```python
from build123d import *

# Parameters (mm, degrees)
F1_DEPTH = 43.942
F2_DEPTH = 1.5875


with BuildPart() as f1:
    # F0 (on Front) → F1 (new body)
    with BuildSketch(Plane.XZ):
        with BuildLine():
            Line((-187.452, 109.982), (-187.452, -109.982))
            Line((-187.452, -109.982), (-100.33, -109.982))
            Line((-100.33, -109.982), (-87.630004, -109.982))
            Line((-87.630004, -109.982), (-0.060038, -109.982))
            ThreePointArc((-0.060038, -109.982), (0, -109.981677), (0.060038, -109.982))
            Line((0.060038, -109.982), (87.630004, -109.982))
            Line((87.630004, -109.982), (100.33, -109.982))
            Line((100.33, -109.982), (187.452, -109.982))
            Line((187.452, -109.982), (187.452, 109.982))
            Line((187.452, 109.982), (100.33, 109.982))
            Line((100.33, 109.982), (87.630004, 109.982))
            Line((87.630004, 109.982), (0.060038, 109.982))
            ThreePointArc((0.060038, 109.982), (0, 109.981677), (-0.060038, 109.982))
            Line((-0.060038, 109.982), (-87.630004, 109.982))
            Line((-87.630004, 109.982), (-100.33, 109.982))
            Line((-100.33, 109.982), (-187.452, 109.982))
        make_face()
    extrude(amount=F1_DEPTH)

    # F0 (on Front) → F2 (join)
    with BuildSketch(Plane.XZ):
        with BuildLine():
            Line((-187.452, 123.952), (-187.452, 109.982))
            Line((-187.452, 109.982), (-100.33, 109.982))
            Line((-100.33, 109.982), (-100.33, 123.952))
            Line((-100.33, 123.952), (-120.4341, 123.952))
            Line((-120.4341, 123.952), (-120.4341, 119.612701))
            Line((-120.4341, 119.612701), (-120.4341, 119.579099))
            ThreePointArc((-120.4341, 119.579099), (-122.428, 117.601929), (-124.4219, 119.579099))
            Line((-124.4219, 119.579099), (-124.4219, 123.952))
            Line((-124.4219, 123.952), (-160.5661, 123.952))
            Line((-160.5661, 123.952), (-160.5661, 119.612701))
            Line((-160.5661, 119.612701), (-160.5661, 119.579099))
            ThreePointArc((-160.5661, 119.579099), (-161.15005, 118.18595), (-162.543199, 117.602))
            Line((-162.543199, 117.602), (-162.576801, 117.602))
            ThreePointArc((-162.576801, 117.602), (-163.96995, 118.18595), (-164.5539, 119.579099))
            Line((-164.5539, 119.579099), (-164.5539, 123.952))
            Line((-164.5539, 123.952), (-187.452, 123.952))
        make_face()
        with BuildLine():
            Line((-187.452, -109.982), (-187.452, -123.952))
            Line((-187.452, -123.952), (-164.5539, -123.952))
            Line((-164.5539, -123.952), (-164.5539, -119.579099))
            ThreePointArc((-164.5539, -119.579099), (-162.56, -117.601929), (-160.5661, -119.579099))
            Line((-160.5661, -119.579099), (-160.5661, -119.612701))
            Line((-160.5661, -119.612701), (-160.5661, -123.952))
            Line((-160.5661, -123.952), (-124.4219, -123.952))
            Line((-124.4219, -123.952), (-124.4219, -119.579099))
            ThreePointArc((-124.4219, -119.579099), (-122.428, -117.601929), (-120.4341, -119.579099))
            Line((-120.4341, -119.579099), (-120.4341, -119.612701))
            Line((-120.4341, -119.612701), (-120.4341, -123.952))
            Line((-120.4341, -123.952), (-100.33, -123.952))
            Line((-100.33, -123.952), (-100.33, -109.982))
            Line((-100.33, -109.982), (-187.452, -109.982))
        make_face()
        with BuildLine():
            ThreePointArc((5.588, 115.509962), (3.951541, 111.618459), (0.060038, 109.982))
            Line((0.060038, 109.982), (87.630004, 109.982))
            Line((87.630004, 109.982), (87.630004, 123.952))
            Line((87.630004, 123.952), (67.5259, 123.952))
            Line((67.5259, 123.952), (67.5259, 119.579099))
            ThreePointArc((67.5259, 119.579099), (65.532, 117.601929), (63.5381, 119.579099))
            Line((63.5381, 119.579099), (63.5381, 119.612701))
            Line((63.5381, 119.612701), (63.5381, 123.952))
            Line((63.5381, 123.952), (27.3939, 123.952))
            Line((27.3939, 123.952), (27.3939, 119.579099))
            ThreePointArc((27.3939, 119.579099), (25.4, 117.601929), (23.4061, 119.579099))
            Line((23.4061, 119.579099), (23.4061, 119.612701))
            Line((23.4061, 119.612701), (23.4061, 123.952))
            Line((23.4061, 123.952), (5.588, 123.952))
            Line((5.588, 123.952), (5.588, 115.630038))
            ThreePointArc((5.588, 115.630038), (5.588323, 115.57), (5.588, 115.509962))
        make_face()
        with BuildLine():
            Line((187.452, -109.982), (100.33, -109.982))
            Line((100.33, -109.982), (100.33, -123.952))
            Line((100.33, -123.952), (120.4341, -123.952))
            Line((120.4341, -123.952), (120.4341, -119.612701))
            ThreePointArc((120.4341, -119.612701), (120.434029, -119.5959), (120.4341, -119.579099))
            ThreePointArc((120.4341, -119.579099), (122.428, -117.601929), (124.4219, -119.579099))
            Line((124.4219, -119.579099), (124.4219, -123.952))
            Line((124.4219, -123.952), (160.5661, -123.952))
            Line((160.5661, -123.952), (160.5661, -119.612701))
            ThreePointArc((160.5661, -119.612701), (160.566029, -119.5959), (160.5661, -119.579099))
            ThreePointArc((160.5661, -119.579099), (162.56, -117.601929), (164.5539, -119.579099))
            Line((164.5539, -119.579099), (164.5539, -123.952))
            Line((164.5539, -123.952), (187.452, -123.952))
            Line((187.452, -123.952), (187.452, -109.982))
        make_face()
        with BuildLine():
            Line((-87.630004, 123.952), (-87.630004, 109.982))
            Line((-87.630004, 109.982), (-0.060038, 109.982))
            ThreePointArc((-0.060038, 109.982), (-3.951541, 111.618459), (-5.588, 115.509962))
            ThreePointArc((-5.588, 115.509962), (-5.588323, 115.57), (-5.588, 115.630038))
            Line((-5.588, 115.630038), (-5.588, 123.952))
            Line((-5.588, 123.952), (-23.4061, 123.952))
            Line((-23.4061, 123.952), (-23.4061, 119.612701))
            ThreePointArc((-23.4061, 119.612701), (-23.406029, 119.5959), (-23.4061, 119.579099))
            ThreePointArc((-23.4061, 119.579099), (-25.4, 117.601929), (-27.3939, 119.579099))
            Line((-27.3939, 119.579099), (-27.3939, 123.952))
            Line((-27.3939, 123.952), (-63.5381, 123.952))
            Line((-63.5381, 123.952), (-63.5381, 119.612701))
            ThreePointArc((-63.5381, 119.612701), (-63.538029, 119.5959), (-63.5381, 119.579099))
            ThreePointArc((-63.5381, 119.579099), (-65.532, 117.601929), (-67.5259, 119.579099))
            Line((-67.5259, 119.579099), (-67.5259, 123.952))
            Line((-67.5259, 123.952), (-87.630004, 123.952))
        make_face()
        with BuildLine():
            Line((-0.060038, -109.982), (-87.630004, -109.982))
            Line((-87.630004, -109.982), (-87.630004, -123.952))
            Line((-87.630004, -123.952), (-67.5259, -123.952))
            Line((-67.5259, -123.952), (-67.5259, -119.579099))
            ThreePointArc((-67.5259, -119.579099), (-65.532, -117.601929), (-63.5381, -119.579099))
            Line((-63.5381, -119.579099), (-63.5381, -119.612701))
            Line((-63.5381, -119.612701), (-63.5381, -123.952))
            Line((-63.5381, -123.952), (-27.3939, -123.952))
            Line((-27.3939, -123.952), (-27.3939, -119.579099))
            ThreePointArc((-27.3939, -119.579099), (-25.4, -117.601929), (-23.4061, -119.579099))
            Line((-23.4061, -119.579099), (-23.4061, -119.612701))
            Line((-23.4061, -119.612701), (-23.4061, -123.952))
            Line((-23.4061, -123.952), (-5.588, -123.952))
            Line((-5.588, -123.952), (-5.588, -115.630038))
            ThreePointArc((-5.588, -115.630038), (-5.588323, -115.57), (-5.588, -115.509962))
            ThreePointArc((-5.588, -115.509962), (-3.951541, -111.618459), (-0.060038, -109.982))
        make_face()
        with BuildLine():
            Line((87.630004, -109.982), (0.060038, -109.982))
            ThreePointArc((0.060038, -109.982), (3.951541, -111.618459), (5.588, -115.509962))
            ThreePointArc((5.588, -115.509962), (5.588323, -115.57), (5.588, -115.630038))
            Line((5.588, -115.630038), (5.588, -123.952))
            Line((5.588, -123.952), (23.4061, -123.952))
            Line((23.4061, -123.952), (23.4061, -119.612701))
            ThreePointArc((23.4061, -119.612701), (23.406029, -119.5959), (23.4061, -119.579099))
            ThreePointArc((23.4061, -119.579099), (25.4, -117.601929), (27.3939, -119.579099))
            Line((27.3939, -119.579099), (27.3939, -123.952))
            Line((27.3939, -123.952), (63.5381, -123.952))
            Line((63.5381, -123.952), (63.5381, -119.612701))
            ThreePointArc((63.5381, -119.612701), (63.538029, -119.5959), (63.5381, -119.579099))
            ThreePointArc((63.5381, -119.579099), (65.532, -117.601929), (67.5259, -119.579099))
            Line((67.5259, -119.579099), (67.5259, -123.952))
            Line((67.5259, -123.952), (87.630004, -123.952))
            Line((87.630004, -123.952), (87.630004, -109.982))
        make_face()
        with BuildLine():
            Line((100.33, 123.952), (100.33, 109.982))
            Line((100.33, 109.982), (187.452, 109.982))
            Line((187.452, 109.982), (187.452, 123.952))
            Line((187.452, 123.952), (164.5539, 123.952))
            Line((164.5539, 123.952), (164.5539, 119.579099))
            ThreePointArc((164.5539, 119.579099), (162.56, 117.601929), (160.5661, 119.579099))
            Line((160.5661, 119.579099), (160.5661, 119.612701))
            Line((160.5661, 119.612701), (160.5661, 123.952))
            Line((160.5661, 123.952), (124.4219, 123.952))
            Line((124.4219, 123.952), (124.4219, 119.579099))
            ThreePointArc((124.4219, 119.579099), (122.428, 117.601929), (120.4341, 119.579099))
            Line((120.4341, 119.579099), (120.4341, 119.612701))
            Line((120.4341, 119.612701), (120.4341, 123.952))
            Line((120.4341, 123.952), (100.33, 123.952))
        make_face()
    extrude(amount=F2_DEPTH)


solid = f1.part
```
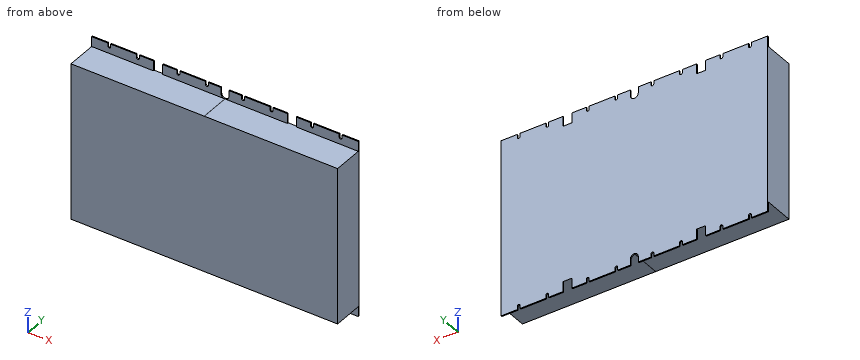
Check sheet for the modelled part. Datum: model origin and axes. Units: mm. Coordinates: 2 decimals unless noted, no trailing zeros. Order: outer loops, then holes, each group sorted by start corner. A loop starts at its lowest first (then second) coordinate and runs counter-clockwise, first axis right, second up. Notation, with made-up numbers: (35, 57) -> (81, 57) arc R23 cw to (81, 69) -> close; hole circle Ø3 at (47, 24). An arc over 180 degrees is marked (long way). Write each question's results on one line, items separated by ' | '. Start each with the question number.
1) Section check A-A (x = -134). Enter the section's corners in (y, z).
2) Depth check by flat-ended pin: pin 1 (4 mm diameter, centred on x = 143, y = -38, fed in from +Z); pin 2 (12 mm diameter, centred on x = 39.5, y = -24.5, fed in from -Z); pin 3 (4 mm diameter, centred on x = 139, z = 115.5, fed in from -Y). Enter the tip coordinate at first touch or a pass-through.
3) Material ranges on line 1 along Z through (x, y) = (88, -6), recorded low to high.
4) Section check B-B (y = -39). Enter the section's corners in (x, z), and give its area (3 significant figures).
Checked values:
1) outline: (-43.94, -109.98) -> (-1.59, -109.98) -> (-1.59, -123.95) -> (0, -123.95) -> (0, 123.95) -> (-1.59, 123.95) -> (-1.59, 109.98) -> (-43.94, 109.98) -> close
2) pin 1: z = 109.98 | pin 2: z = -109.98 | pin 3: y = -1.59
3) line 1: -109.98 to 109.98
4) outline: (-187.45, -109.98) -> (-0.06, -109.98) arc R5.58 cw to (0.06, -109.98) -> (187.45, -109.98) -> (187.45, 109.98) -> (0.06, 109.98) arc R5.58 cw to (-0.06, 109.98) -> (-187.45, 109.98) -> close | area: 82,500 mm²
